Print and shaded views of the part. All mm, measured from the part's lowest x, y and z. A direction names the side the tool comes from. Give positions to 0.01 mm unless a question says otherwise; leave off trailing zeros. Loops run counter-clockwise (first coordinate to the right, second up) from the corner with the lowest first, then second, coordinate; pieces in that order, holes last. Notation, with made-up numbers: M -35.75,21 L 14.25,21 A8 ccw 14.25,32 Z; hole C 77.5,0.25 d3. An arc over 180 degrees is marked long. Answer in a Markdown table with one row per item.
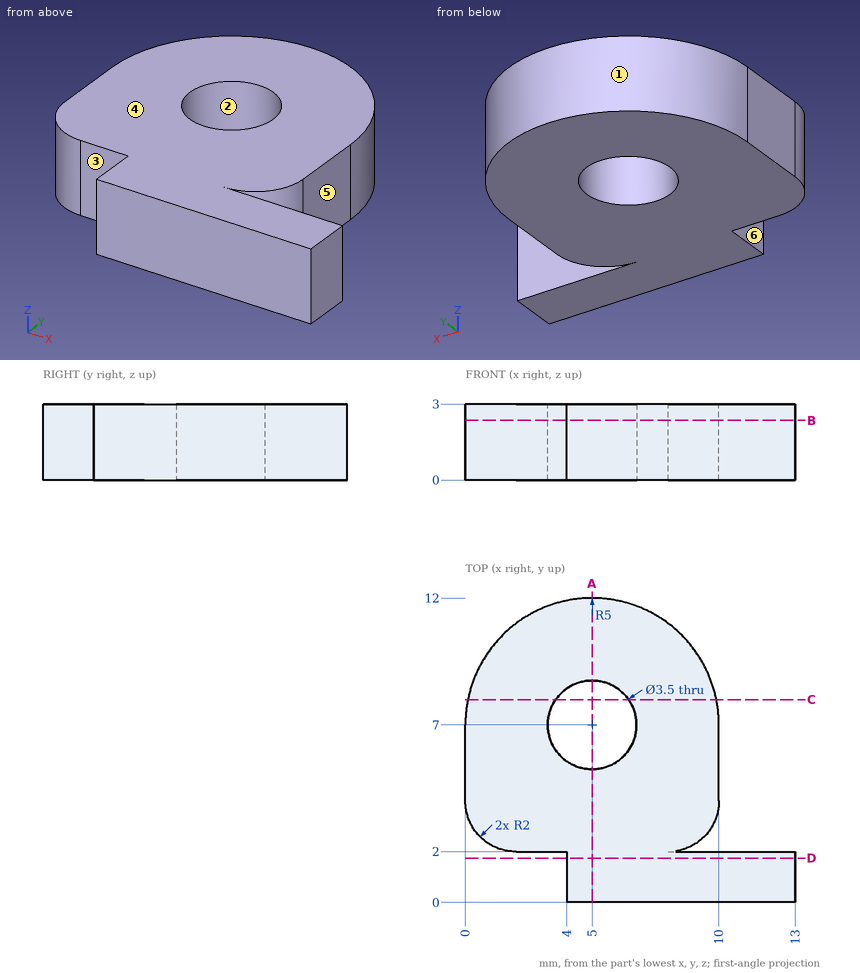
(1) Saw through at C-C, the plane y = 8. Give the cut face in (x, z), and give its area (3 significant figures).
Established:
| item | result |
|---|---|
| outline | M 0.1,0 L 3.56,0 L 3.56,3 L 0.1,3 Z; M 6.44,0 L 9.9,0 L 9.9,3 L 6.44,3 Z |
| area | 20.8 mm2 |
(2) Mould opens along Y. For the marked faces 1, 2 and 3 say: pulls with the +Y half, pulls with the -Y half, needs draft (parallel to the pull), parting line crosses it, or undercut.
Established:
| item | result |
|---|---|
| face 1 | pulls with the +Y half |
| face 2 | undercut |
| face 3 | pulls with the -Y half |
(3) Wall check: L1, parallel to X at y = 7, z = 2.3; L2, parallel to Y at x = 5, z = 2; L3, parallel to X at y = 5, z = 0.25. Give the ranges that are in metal, low to high.
Established:
| item | result |
|---|---|
| L1 | x = 0 to 3.25, 6.75 to 10 |
| L2 | y = 0 to 5.25, 8.75 to 12 |
| L3 | x = 0 to 10 |
(4) Saw through at D-D, the plane y = 1.75. Give the cut face in (x, z), and give its area (3 significant figures).
Established:
| item | result |
|---|---|
| outline | M 4,0 L 13,0 L 13,3 L 4,3 Z |
| area | 27.0 mm2 |
(5) Which spindle directions (+Z, -Z, +X, -X, +Y, -Y) get a long thin tool onto all of the face, cutting with end or side? Do the marked faces 4, 5 and 6. Say none if no direction does.
Established:
| item | result |
|---|---|
| face 4 | +Z, +X, -X, +Y, -Y |
| face 5 | +Z, -Z, +X, +Y |
| face 6 | +Z, -Z, -X, -Y |
(6) Saw through at B-B, the plane z = 2.35. Give the cut face in (x, y), and give its area (3 significant figures).
Established:
| item | result |
|---|---|
| outline | M 0,4 A2 ccw 2,2 L 4,2 L 4,0 L 13,0 L 13,2 L 8,2 A2 ccw 10,4 L 10,7 A5 ccw 0,7 Z; hole C 5,7 d3.5 |
| area | 95.9 mm2 |
(7) Saw through at A-A, the plane x = 5. Give the cut face in (y, z), and give its area (3 significant figures).
Established:
| item | result |
|---|---|
| outline | M 0,0 L 5.25,0 L 5.25,3 L 0,3 Z; M 8.75,0 L 12,0 L 12,3 L 8.75,3 Z |
| area | 25.5 mm2 |
(8) Flat gauge pins, fed straight in: P1, Ø1, axis at y = 10.5, z = 2, coming from the -X side; P2, Ø1.5, axis at x = 10, z = 1.5, coming from the +Y side; P3, Ø1.5, axis at y = 8, z = 2, coming from the +X side; P4, Ø1, axis at x = 8.5, y = 1.5, coming from the -Z side. Where does each tip first touch, or does it go through?
Established:
| item | result |
|---|---|
| P1 | stops at x = 1 |
| P2 | stops at y = 9.63 |
| P3 | stops at x = 9.99 |
| P4 | stops at z = 0 |
